Geometry check sheet. Reference: drawing and pictorial views, mm from the part's lowest x, y, z. A direction names the side the tool comes from. Coordinates: 2 decimals unless noted, no trailing zeros. Loops run counter-clockwise (first coordinate to the right, second up) from the corner with the lowest first, then second, coordinate; pieces in that order, holes last. Notation, with made-up numbers: (70.25, -34) -> (124.25, -34) arc R30 ccw to (124.25, 3) -> close; hole circle Ø8 at (86, -2.5). An arc over 180 degrees is marked (long way). Use CSV: the item, a comma, the result in double quotes.
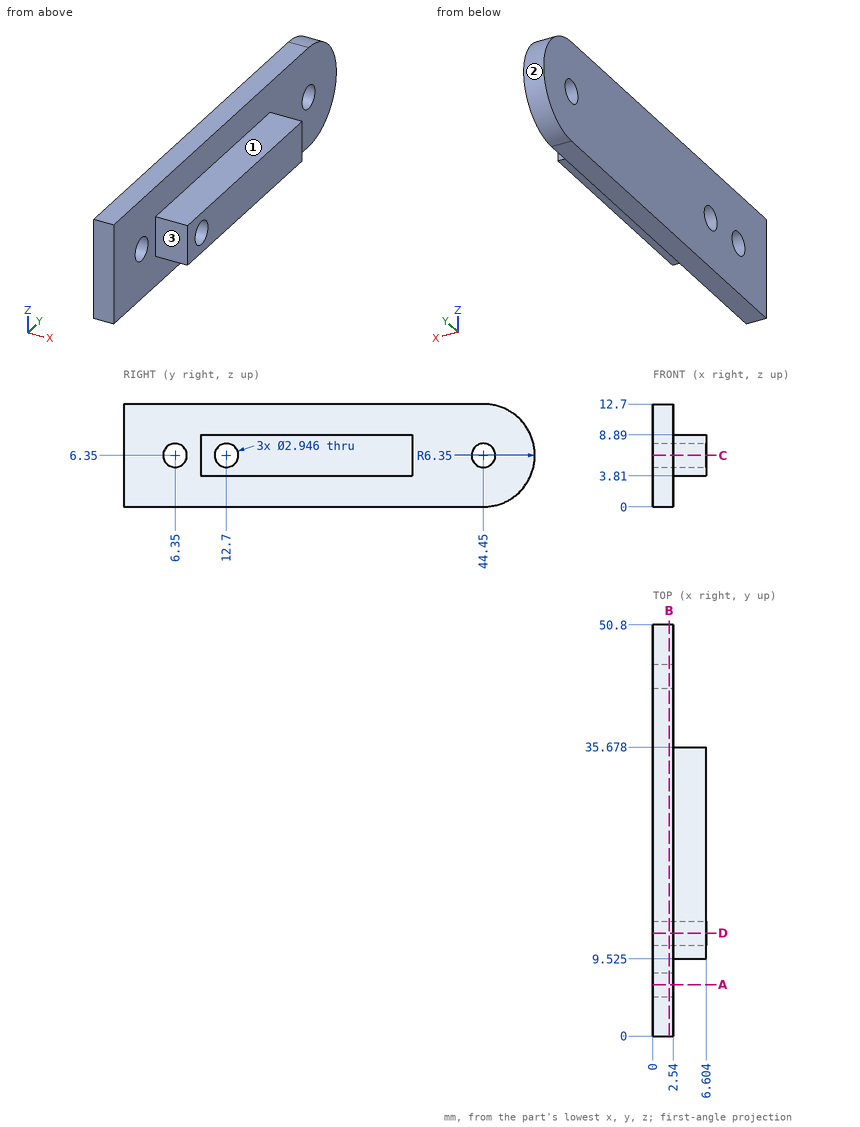
1) Cross-section at A-A on y = 6.35. Record the boundary of the cut face in (x, z).
Answer below:
outline,"(0, 0) -> (2.54, 0) -> (2.54, 4.88) -> (0, 4.88) -> close; (0, 7.82) -> (2.54, 7.82) -> (2.54, 12.7) -> (0, 12.7) -> close"
2) Cross-section at C-C on z = 6.35. Record the boundary of the cut face in (x, y) (1 decimal), and give its area (3 significant figures).
Answer below:
outline,"(0, 0) -> (2.5, 0) -> (2.5, 4.9) -> (0, 4.9) -> close; (0, 7.8) -> (2.5, 7.8) -> (2.5, 9.5) -> (6.6, 9.5) -> (6.6, 11.2) -> (0, 11.2) -> close; (0, 14.2) -> (6.6, 14.2) -> (6.6, 35.7) -> (2.5, 35.7) -> (2.5, 43) -> (0, 43) -> close; (0, 45.9) -> (2.5, 45.9) -> (2.5, 50.8) -> (0, 50.8) -> close"
area,"201 mm²"
3) Cross-section at D-D on y = 12.7. Record the boundary of the cut face in (x, z).
Answer below:
outline,"(0, 0) -> (2.54, 0) -> (2.54, 3.81) -> (6.6, 3.81) -> (6.6, 4.88) -> (0, 4.88) -> close; (0, 7.82) -> (6.6, 7.82) -> (6.6, 8.89) -> (2.54, 8.89) -> (2.54, 12.7) -> (0, 12.7) -> close"
4) Thickness scan on line 1 along Z through (x, y) = (0.85, 44.45); line 2 along Y through (x, z) = (1.4, 6.35); line 3 along Y through (x, z) = (2.75, 6.35) (1 decimal). Record the ranges inside material, lowest first. Write a range as from..to.
Answer below:
line 1,"z = 0..4.88, 7.82..12.7"
line 2,"y = 0..4.88, 7.82..11.23, 14.17..42.98, 45.92..50.8"
line 3,"y = 9.5..11.2, 14.2..35.7"
5) Access from +Z, -Z, +X, -X, +Y, -Y to the whole of each face (thin tool, end or side, straight path). Record for the marked faces 1, 2 and 3.
Answer below:
face 1,"+Z, +X, +Y, -Y"
face 2,"+X, -X, +Y"
face 3,"+Z, -Z, +X, -Y"
6) Cross-section at B-B on x = 2. Record the boundary of the cut face in (y, z).
Answer below:
outline,"(0, 0) -> (44.45, 0) arc R6.35 ccw to (44.45, 12.7) -> (0, 12.7) -> close; hole circle Ø2.95 at (6.35, 6.35); hole circle Ø2.95 at (12.7, 6.35); hole circle Ø2.95 at (44.45, 6.35)"
7) Go/stop test with flat-tipped pins: pin 1 Ø2 at (x, z) = (4.5, 7.5) entering from +Y; pin 2 Ø1 at (x, z) = (1, 8.5) entering from +Y; pin 3 Ø2 at (x, z) = (4, 5) entering from -Y (3 decimals); pin 4 Ø1.8 at (y, z) = (44.45, 6.35) entering from +X. Record where each tip stops, or that it passes through.
Answer below:
pin 1,"stops at y = 35.68"
pin 2,"stops at y = 50.58"
pin 3,"stops at y = 9.525"
pin 4,"passes through"
